Autodesk Inventor part; units mm, degrees
ref_plane "YZ Plane" through (0, 0, 0) normal (1, 0, 0) x (0, 1, 0)
ref_plane "XZ Plane" through (0, 0, 0) normal (0, 1, 0) x (-1, 0, 0)
ref_plane "XY Plane" through (0, 0, 0) normal (0, 0, 1) x (1, 0, 0)
sketch "Sketch1" plane through (0, 0, 0) normal (0, 0, 1) x (1, 0, 0)
  line L0 (0, 0) -> (165.1, 0)
  line L1 (165.1, 0) -> (165.1, 12.7)
  line L2 (165.1, 12.7) -> (0, 12.7)
  line L3 (0, 12.7) -> (0, 0)
  line L4 (165.1, 0) -> (165.1, -12.7)
  line L5 (165.1, -12.7) -> (0, -12.7)
  line L6 (0, -12.7) -> (0, 0)
  dimension "d2" = 165.1
  dimension "d3" = 25.4
extrude "Extrusion1" add sketch "Sketch1" along normal mid plane 31.75
sketch "Sketch3" plane through (0, 12.7, 15.875) normal (0, 1, 0) x (1, 0, 0)
  line L0 (0, 15.875) -> (165.1, 15.875) construction
  line L1 (165.1, 31.75) -> (165.1, 0) construction
  line L2 (0, 31.75) -> (0, 0)
  line L3 (0, 23.495) -> (139.7, 23.495)
  line L4 (139.7, 23.495) -> (139.7, 15.875)
  line L5 (0, 23.495) -> (0, 15.875)
  line L6 (0, 0) -> (0, 31.75)
  line L7 (0, 8.255) -> (139.7, 8.255)
  line L8 (139.7, 8.255) -> (139.7, 15.875)
  dimension "d6" = 139.7
  dimension "d7" = 7.62
extrude "Extrusion2" cut sketch "Sketch3" against normal through all
sketch "Sketch4" plane through (0, 0, 15.875) normal (0, 0, 1) x (1, 0, 0)
  circle A0 centre (12.7, 0) radius 5.3975
  circle A1 centre (152.4, 0) radius 5.3975
  line L0 (165.1, -12.7) -> (165.1, 12.7)
  point P0 (0, 0)
  dimension "d10" = 10.795
  dimension "d11" = 12.7
  dimension "d12" = 12.7
extrude "Extrusion3" cut sketch "Sketch4" against normal through all
properties part number "connectiingRodV03"
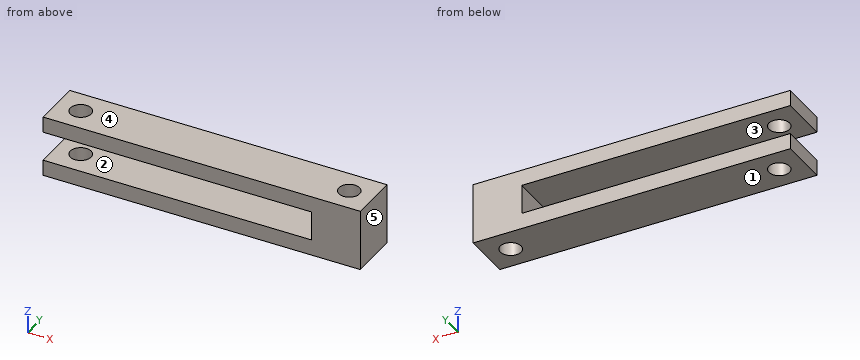
Verification items for the finished model (mm, model axes). Face numbers are marked on the shaded views. A direction names the side the tool comes from. Coordinates: 2 decimals unless noted, no trailing zeros. Loops run counter-clockwise (first coordinate to the right, second up) from the corner with the lowest first, then second, coordinate; pieces in that order, holes last. Notation, with made-up numbers: (-14.75, 73.5) - (-3.75, 73.5) arc R18 ccw to (-3.75, 99.5) - close; hole circle Ø4 at (-16.75, 78). An arc over 180 degrees is marked (long way). Answer as a JSON object with one key per item and string values.
(1) Mould release check, pull along Z, two halves, no side actions. Record for the marked faces 3, 4 and 5: pulls with the +Z half, pulls with the -Z half, needs draft (parallel to the pull), parting line crosses it, or undercut.
Response:
{"face 3": "undercut", "face 4": "pulls with the +Z half", "face 5": "needs draft"}
(2) Cross-section at B-B, the plane y = 0. Record the boundary of the cut face in (x, z) (1 decimal).
Response:
{"outline": "(0, -15.9) - (7.3, -15.9) - (7.3, -7.6) - (0, -7.6) - close; (0, 7.6) - (7.3, 7.6) - (7.3, 15.9) - (0, 15.9) - close; (18.1, -15.9) - (147, -15.9) - (147, 15.9) - (18.1, 15.9) - (18.1, 7.6) - (139.7, 7.6) - (139.7, -7.6) - (18.1, -7.6) - close; (157.8, -15.9) - (165.1, -15.9) - (165.1, 15.9) - (157.8, 15.9) - close"}
(3) Access from +Z, -Z, +X, -X, +Y, -Y to the whole of each face (thin tool, end or side, straight path). Record for the marked faces 1 and 2.
Response:
{"face 1": "-Z, +X, -X, +Y, -Y", "face 2": "-X, +Y, -Y"}
(4) Cross-section at D-D, the plane x = 90.5. Record the boundary of the cut face in (y, z) (3 decimals).
Response:
{"outline": "(-12.7, -15.875) - (12.7, -15.875) - (12.7, -7.62) - (-12.7, -7.62) - close; (-12.7, 7.62) - (12.7, 7.62) - (12.7, 15.875) - (-12.7, 15.875) - close"}
(5) Cross-section at C-C, the plane z = -1. Record the boundary of the cut face in (x, y) (1 decimal).
Response:
{"outline": "(139.7, -12.7) - (165.1, -12.7) - (165.1, 12.7) - (139.7, 12.7) - close; hole circle Ø10.8 at (152.4, 0)"}
(6) Scan lines: line 1 along Y through (x, z) = (153, 14.5); line 2 along Z through (x, y) = (35, 0.5) (3 decimals); line 3 along X through (y, z) = (6, -6). Record each from-to range of solid material in increasing order.
Response:
{"line 1": "y = -12.7 to -5.36, 5.36 to 12.7", "line 2": "z = -15.875 to -7.62, 7.62 to 15.875", "line 3": "x = 139.7 to 165.1"}
(7) Cross-section at A-A, the plane x = 12.7. Record the boundary of the cut face in (y, z) (1 decimal), then the cut area to 3 significant figures.
Response:
{"outline": "(-12.7, -15.9) - (-5.4, -15.9) - (-5.4, -7.6) - (-12.7, -7.6) - close; (-12.7, 7.6) - (-5.4, 7.6) - (-5.4, 15.9) - (-12.7, 15.9) - close; (5.4, -15.9) - (12.7, -15.9) - (12.7, -7.6) - (5.4, -7.6) - close; (5.4, 7.6) - (12.7, 7.6) - (12.7, 15.9) - (5.4, 15.9) - close", "area": "241 mm²"}
(8) Go/stop test with flat-tipped pins: pin 1 Ø8.5 at (x, y) = (12.7, 0) entering from +Z; pin 2 Ø10 at (y, z) = (1.5, 3) entering from -X; pin 3 Ø12 at (y, z) = (-2, 0) entering from -X. Record where each tip stops, or that it passes through.
Response:
{"pin 1": "passes through", "pin 2": "stops at x = 0", "pin 3": "stops at x = 139.7"}
